Geometry check sheet. Reference: the model listing, model coordinates, mm. A direction names the side the tool comes from. Round coordinates to 2 decimals unless told otherwise and drop trailing zeros. Write each loop counter-clockwise with the first axis right and the second up, starting at its lowest first coordinate (ties: lowest second). Pieces come first, ordered by that corner, then holes. Notation, with made-up numbers: M 55.5,-38 L 105.5,-38 A25 ccw 105.5,-17 Z; hole C 32,33.5 d11. An arc over 180 degrees is marked long. Put each result on its own line as item: value. Start each with the question number.
(1) Section check D-D on x = 0.25. Record the cut outline in (y, z).
(2) Tool access check on faces 3 (the flat face through (0, 0, 0)), 4 (the flat face through (1, 0, 0)). Record the directions out of +Z, -Z, +X, -X, +Y, -Y that give a thin tool (end or side, any length) a straight path to the whole face; none if there is none.
(3) Gauge pin test, flat ends, axial feed: pin 1 (4 mm diameter, centred on y = 0.5, z = -1, fed in from -X); pin 2 (1.5 mm diameter, centred on x = -2.5, z = -1.5, fed in from +Y). Record the tip position at first contact, or that the pin passes through.
(4) Section check A-A on z = 0. Record the cut outline in (x, y).
(5) Section check C-C on x = -1.25. Record the cut outline in (y, z), then the cut area to 3 significant figures.
(6) Material ranges on probe 1 along Y at (x, z) = (-1.5, 0); probe 2 along Y at (x, z) = (-2.5, -2); probe 3 along X at (y, z) = (1.25, 1.25), recorded low to high.
(7) Mould release check, pull along Z, two halves, no side actions. Record for faces 1 (the flat face through (-3.25, -3, 0)), 2 (the flat face through (-2, -2.157, 0)): pulls with the +Z half, pulls with the -Z half, needs draft (parallel to the pull), parting line crosses it, or undercut.
(8) Section check B-B on y = 0. Record the cut outline in (x, z), then the cut area to 3 significant figures.
from build123d import *

# Parameters (mm, degrees)
SKETCH1_R           = 4
BOSS_EXTRUDE1_DEPTH = 3.25
SKETCH2_R           = 4
BOSS_EXTRUDE2_DEPTH = 1


with BuildPart() as part:
    # Sketch1 → Boss-Extrude1 (new body)
    with BuildSketch(Plane(origin=(0, 0, 0), x_dir=(0, 0, -1), z_dir=(1, 0, 0))):
        Circle(SKETCH1_R)
        with BuildLine():
            Line((-1.527350647, -2.157), (1.527350647, -2.157))
            ThreePointArc((1.527350647, -2.157), (0, 2.643), (-1.527350647, -2.157))
        make_face(mode=Mode.SUBTRACT)
    extrude(amount=-BOSS_EXTRUDE1_DEPTH)

    # Sketch2 → Boss-Extrude2 (add)
    with BuildSketch(Plane(origin=(0, 0, 0), x_dir=(0, 0, -1), z_dir=(1, 0, 0))):
        Circle(SKETCH2_R)
    extrude(amount=BOSS_EXTRUDE2_DEPTH)


solid = part.part
Answers follow:
1. outline: C 0,0 d8
2. face 3: -X
2. face 4: +Z, -Z, +X, +Y, -Y
3. pin 1: stops at x = -3.25
3. pin 2: stops at y = 3.93
4. outline: M -3.25,-4 L 1,-4 L 1,4 L -3.25,4 L -3.25,2.64 L 0,2.64 L 0,-2.16 L -3.25,-2.16 Z
5. outline: C 0,0 d8; hole M -2.16,-1.53 A2.64 ccw long -2.16,1.53 Z
5. area: 29.3 mm^2
6. probe 1: y = -4 to -2.16, 2.64 to 4
6. probe 2: y = -3.46 to -1.73, 1.73 to 3.46
6. probe 3: x = 0 to 1
7. face 1: needs draft
7. face 2: undercut
8. outline: M -3.25,-4 L 1,-4 L 1,4 L -3.25,4 L -3.25,2.64 L 0,2.64 L 0,-2.64 L -3.25,-2.64 Z
8. area: 16.8 mm^2
